Verification items for the finished model (mm, model axes). A direction names the side the tool comes from. Round coordinates to 2 decimals unless told otherwise and drop trailing zeros. Write each loop counter-clockwise with the first axis right and the second up, starting at its lowest first coordinate (ties: lowest second). Pieces come first, ordered by that corner, then holes. Notation, with made-up numbers: M 69.5,-18.5 L 100.5,-18.5 A21 ccw 100.5,-12.5 Z; hole C 47.25,-26.75 d3. An arc over 180 degrees is marked long. Answer in a Markdown table with one row per item. Add a question column.
1. Sectioned sample at B-B on y = -21.5. Record the cut outline in (x, z), plus the area to 3 significant figures.
2. Go/stop test with flat-tipped pins: pin 1 Ø11 at (x, y) = (19.5, -18.5) entering from +Z; pin 2 Ø1.5 at (x, y) = (13.5, -6.5) entering from -Z; pin 3 Ø4 at (x, y) = (19, -12) entering from +Z. Record where each tip stops, or that it passes through.
3. Set-up check for faces 5 (the flat face through (13, -3, -5)), 6 (the flat face through (3.281, -12, 2)), 7 (the flat face through (13, -20, -17)), 8 (the cylindrical face through (10.05, -22.46, -13.3)): record each of +Z, -Z, +X, -X, +Y, -Y from which the full face is reachable in a straight line by a thin tool's end or side.
4. Sectioned sample at D-D on y = -14.75. Record the cut outline in (x, z).
5. Sectioned sample at C-C on x = 7.5. Record the cut outline in (y, z).
6. Sectioned sample at A-A on z = -16. Record the cut outline in (x, y).
7. Material ranges on probe 1 along X at (y, z) = (-19.25, -6.75); probe 2 along Y at (x, z) = (13, -7.5); probe 3 along Z at (x, y) = (-22, -18.75), recorded low to high.
8. Draft check along X on faces 1 (the flat face through (0, 0, -7)), 2 (the cylindrical face through (-17, -22, -16)), 3 (the flat face through (-19.58, -12.34, -4.14)), 4 (the flat face through (25, -12, -9)). Enter one of: pulls with the +X half, pulls with the -X half, needs draft (parallel to the pull), parting line crosses it, or undercut.
```python
from build123d import *

# Parameters (mm, degrees)
F1_DEPTH = 25
F2_W     = 18.718621
F2_H     = 19
F3_DEPTH = 7
F4_R     = 1
F5_R     = 5
F6_DEPTH = 5
F7_R     = 4
F8_DEPTH = 5


with BuildPart() as f1:
    # F0 (on Front) → F1 (new body)
    with BuildSketch(Plane.XZ):
        Polygon((-25, -5), (-25, -15), (25, -15), (25, -6), (25, -2), (3.281379, -2), (3.281379, 5.433359), (-11.718621, 5.433359), (-15.123117, -3.435655), align=None)
    extrude(amount=F1_DEPTH)

    # F2 (on face) → F3 (cut)
    with BuildSketch(Plane.XY.offset(-2)):
        with Locations((12.64069, -12.5)):
            Rectangle(F2_W, F2_H)
    extrude(amount=-F3_DEPTH, mode=Mode.SUBTRACT)

    # F4
    f4_edges = [f1.edges().sort_by_distance(p)[0] for p in [
        (-20.061558, 0, -4.217828),
        (-20.061558, -25, -4.217828),
        (-25, -12.5, -5),
    ]]
    fillet(f4_edges, radius=F4_R)

    # F5 (on face) → F6 (cut)
    with BuildSketch(Plane.XZ.offset(25)):
        with Locations((-13, -16)):
            Circle(F5_R)
        with Locations((13, -16)):
            Circle(F5_R)
    extrude(amount=-F6_DEPTH, mode=Mode.SUBTRACT)

    # F7 (on face) → F8 (join, through all)
    with BuildSketch(Plane.XZ.offset(20)):
        with Locations((-13, -16)):
            Circle(F7_R)
        with Locations((13, -16)):
            Circle(F7_R)
    extrude(amount=F8_DEPTH)


solid = f1.part
```
Geometry check:
| question | item | result |
|---|---|---|
| 1 | outline | M -25,-15 L -17.9,-15 A5 cw -8.1,-15 L 8.1,-15 A5 cw 17.9,-15 L 25,-15 L 25,-2 L 22,-2 L 22,-9 L 3.28,-9 L 3.28,5.43 L -11.72,5.43 L -15.12,-3.44 L -24.16,-4.87 A1 ccw -25,-5.85 Z; C -13,-16 d8; C 13,-16 d8 |
| 1 | area | 660 mm2 |
| 2 | pin 1 | stops at z = -2 |
| 2 | pin 2 | stops at z = -15 |
| 2 | pin 3 | stops at z = -9 |
| 3 | face 5 | +Z |
| 3 | face 6 | +Z, +X, +Y, -Y |
| 3 | face 7 | -Z, +X, -X, +Y |
| 3 | face 8 | -Y |
| 4 | outline | M -25,-15 L 25,-15 L 25,-2 L 22,-2 L 22,-9 L 3.28,-9 L 3.28,5.43 L -11.72,5.43 L -15.12,-3.44 L -24.16,-4.87 A1 ccw -25,-5.85 Z |
| 5 | outline | M -25,-15 L 0,-15 L 0,-2 L -3,-2 L -3,-9 L -22,-9 L -22,-2 L -25,-2 Z |
| 6 | outline | M -17,-25 L -9,-25 L -9,-20 L -17,-20 Z; M 9,-25 L 17,-25 L 17,-20 L 9,-20 Z |
| 7 | probe 1 | x = -25 to 3.28, 22 to 25 |
| 7 | probe 2 | y = -25 to -22, -3 to 0 |
| 7 | probe 3 | z = -15 to -4.52 |
| 8 | face 1 | needs draft |
| 8 | face 2 | undercut |
| 8 | face 3 | pulls with the -X half |
| 8 | face 4 | pulls with the +X half |
